Autodesk Inventor part; units mm, degrees
ref_plane "YZ Plane" through (0, 0, 0) normal (1, 0, 0) x (0, 1, 0)
ref_plane "XZ Plane" through (0, 0, 0) normal (0, 1, 0) x (-1, 0, 0)
ref_plane "XY Plane" through (0, 0, 0) normal (0, 0, 1) x (1, 0, 0)
sketch "Sketch1" plane through (0, 0, 0) normal (0, 1, 0) x (-1, 0, 0)
  line L0 (0, 0) -> (61.9125, 0)
  line L1 (61.9125, 0) -> (61.9125, -43.18)
  line L2 (61.9125, -43.18) -> (0, -43.18)
  line L3 (0, -43.18) -> (0, 0)
  dimension "d0" = 61.9125
  dimension "d1" = 43.18
extrude "Extrusion1" add sketch "Sketch1" along normal blind 6.35
sketch "Sketch2" plane through (0, 6.35, 0) normal (0, 1, 0) x (1, 0, 0)
  line L0 (-61.9125, 43.18) -> (-61.9125, 0)
  line L1 (-61.9125, 0) -> (0, 0)
  line L2 (0, 0) -> (0, 43.18)
  line L3 (-61.9125, 43.18) -> (0, 43.18)
  line L4 (-61.9125, 43.18) -> (-61.9125, 0)
  line L5 (0, 43.18) -> (-61.9125, 43.18)
  line L6 (-61.9125, 0) -> (0, 0)
  line L7 (0, 0) -> (0, 43.18)
  point P0 (-41.5925, 21.59)
  point P1 (-21.2725, 21.59)
  point P2 (-26.3525, 30.48)
  point P3 (-26.3525, 12.7)
  dimension "d10" = 21.2725
  dimension "d11" = 21.59
  dimension "d14" = 21.59
  dimension "d15" = 20.32
  dimension "d18" = 12.7
  dimension "d19" = 12.7
  dimension "d20" = 15.24
  dimension "d21" = 15.24
hole "Hole1" at (-21.2725, 6.35, -21.59) direction (0, -1, 0) diameter 6.35 depth 10.9728 tip angle 118
hole "Hole2" at (-41.5925, 6.35, -21.59) direction (0, -1, 0) diameter 12.7 end through all
hole "Hole3" at (-26.3525, 6.35, -30.48) at (-26.3525, 6.35, -12.7) direction (0, -1, 0) diameter 5.1054 end through all
sketch "Sketch3" plane through (-61.9125, 0, -43.18) normal (-1, 0, 0) x (0, 0, 1)
  line L0 (43.18, 0) -> (43.18, 6.35)
  line L1 (0, 0) -> (0, 6.35)
  line L2 (0, 0) -> (43.18, 0)
  point P0 (6.35, 3.175)
  point P1 (36.83, 3.175)
  dimension "d50" = 6.35
  dimension "d51" = 6.35
  dimension "d52" = 3.175
hole "Hole4" at (-61.9125, 3.175, -36.83) at (-61.9125, 3.175, -6.35) direction (1, 0, 0) diameter 2.6416 depth 10.9728 tip angle 118
properties part number "AR-BracketRight2"
Build history of the part. All positions in model axes, mm. A direction names the side the tool comes from. Round coordinates to 2 decimals unless told otherwise and drop trailing zeros. Loops run counter-clockwise (first coordinate to the right, second up) from the corner with the lowest first, then second, coordinate; pieces in that order, holes last. Notation, with made-up numbers: (-8.5, 53) -> (24.5, 53) arc R17 cw to (24.5, 76) -> close; hole circle Ø10 at (46, -27). An arc over 180 degrees is marked (long way). One line per item, written item: value. Start each with the question number.
Q1. Cut at A-A on z = -30.48. List the corners of the cut face in (x, y).
Q2. Cut at C-C on z = -21.59. List the corners of the cut face in (x, y).
Q3. Two-plate mould, pull along Z, no slides. Class faces 1 (the face through (-31, 3, -43.18)), 2 (the face through (-61.912, 3, -21)), 3 (the face through (-31, 3, 0)), 4 (the face through (-25.375, 3.131, -28.122)): released by +Z, released by -Z, zero draft, split by the parting line, or undercut.
Q4. Cut at D-D on x = -27. List the corners of the cut face in (y, z), plus the area to 3 significant figures.
Q5. Cut at B-B on x = -45.5. List the corners of the cut face in (y, z), plus the area to 3 significant figures.
Q6. 3-axis set-ups, long thin cutter, end or side, ignore diameter. For faces 5 (the face through (-47.89, 3.13, -22.42)), 6 (the face through (-56.35, 3.68, -5.13)): which of +Z, -Z, +X, -X, +Y, -Y reach the whole face in a straight line?
Q7. Probe line 1 along Y through (x, z) = (-56.5, -36.83); line 2 along X through (y, z) = (4.5, -21.59); line 3 along X through (y, z) = (2.75, -21). List the from-to ranges inside material, lowest first.
Computed:
1. outline: (-61.91, 0) -> (-28.91, 0) -> (-28.91, 6.35) -> (-61.91, 6.35) -> close; (-23.8, 0) -> (0, 0) -> (0, 6.35) -> (-23.8, 6.35) -> close
2. outline: (-61.91, 0) -> (-47.94, 0) -> (-47.94, 6.35) -> (-61.91, 6.35) -> close; (-35.24, 0) -> (-24.45, 0) -> (-24.45, 6.35) -> (-35.24, 6.35) -> close; (-18.1, 0) -> (0, 0) -> (0, 6.35) -> (-18.1, 6.35) -> close
3. face 1: released by -Z
3. face 2: zero draft
3. face 3: released by +Z
3. face 4: undercut
4. outline: (0, -43.18) -> (6.35, -43.18) -> (6.35, -32.95) -> (0, -32.95) -> close; (0, -28.01) -> (6.35, -28.01) -> (6.35, -15.17) -> (0, -15.17) -> close; (0, -10.23) -> (6.35, -10.23) -> (6.35, 0) -> (0, 0) -> close
4. area: 211 mm²
5. outline: (0, -43.18) -> (6.35, -43.18) -> (6.35, -26.6) -> (0, -26.6) -> close; (0, -16.58) -> (6.35, -16.58) -> (6.35, 0) -> (0, 0) -> close
5. area: 211 mm²
6. face 5: +Y, -Y
6. face 6: -X
7. line 1: 0 to 1.85, 4.5 to 6.35
7. line 2: -61.91 to -47.94, -35.24 to -24.45, -18.1 to 0
7. line 3: -61.91 to -47.92, -35.27 to -24.39, -18.15 to 0
